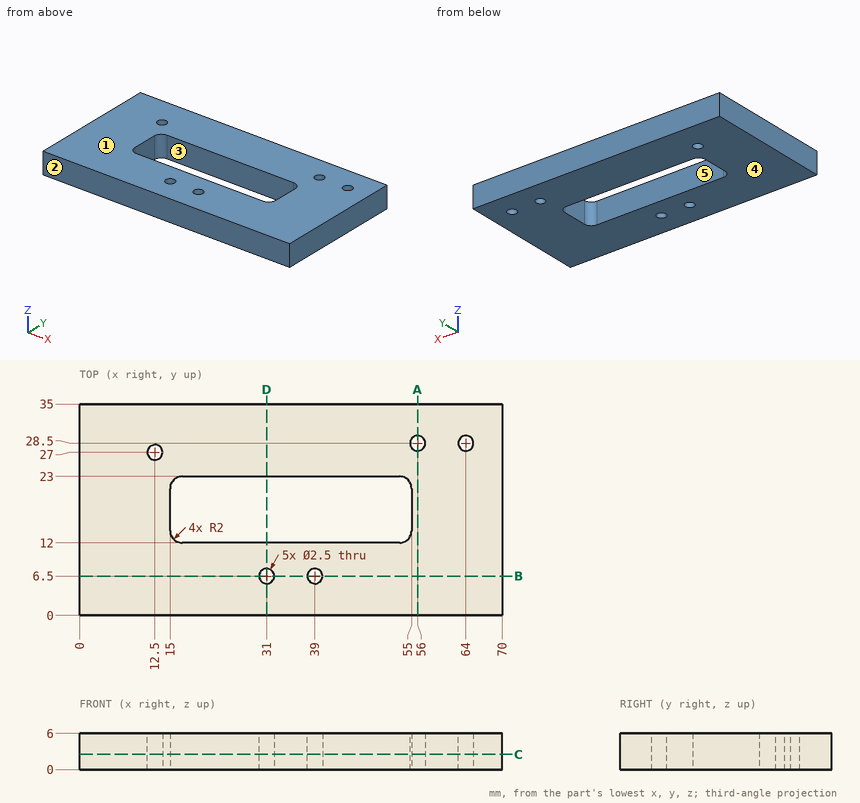
Drawing for the job (mm, zero at the part's lowest x, y, z). A direction names the side the tool comes from. Coordinates: 2 decimals unless noted, no trailing zeros. Order: outer loops, then holes, each group sorted by start corner. A loop starts at its lowest first (then second) coordinate and runs counter-clockwise, first axis right, second up. Notation, with made-up numbers: (28, 55.5) -> (49, 55.5) arc R29 ccw to (49, 90.5) -> close; hole circle Ø2 at (5.5, 65.5). An arc over 180 degrees is marked (long way). Return JSON: item names as keys, results as strings.
Item 1: Mould opens along Y. For the marked faces 1, 2 and 3 say: pulls with the +Y half, pulls with the -Y half, needs draft (parallel to the pull), parting line crosses it, or undercut.
Model answer:
{"face 1": "needs draft", "face 2": "pulls with the -Y half", "face 3": "undercut"}
Item 2: Slice it at C-C (z = 2.5). Write the cut outline in (x, y).
Model answer:
{"outline": "(0, 0) -> (70, 0) -> (70, 35) -> (0, 35) -> close; hole circle Ø2.5 at (12.5, 27); hole (15, 14) arc R2 ccw to (17, 12) -> (53, 12) arc R2 ccw to (55, 14) -> (55, 21) arc R2 ccw to (53, 23) -> (17, 23) arc R2 ccw to (15, 21) -> close; hole circle Ø2.5 at (31, 6.5); hole circle Ø2.5 at (39, 6.5); hole circle Ø2.5 at (56, 28.5); hole circle Ø2.5 at (64, 28.5)"}
Item 3: 3-axis set-ups, long thin cutter, end or side, ignore diameter. For the marked faces 4 and 5: which of +Z, -Z, +X, -X, +Y, -Y reach the whole face in a straight line?
Model answer:
{"face 4": "-Z, +X, -X, +Y, -Y", "face 5": "+Z, -Z"}
Item 4: Pin check, flat tips, straight feed: P1, Ø2, axis at x = 56, y = 28.5, coming from the +Z side; P2, Ø3, axis at x = 64, y = 28.5, coming from the +Z side. Stop position of each tip, or through.
Model answer:
{"P1": "passes through", "P2": "stops at z = 6"}
Item 5: Wall check: line 1 along Y through (x, z) = (31, 3.7); line 2 along X through (y, z) = (7, 1.5); line 3 along Y through (x, z) = (24.5, 0.75). Give the ranges that are in metal, low to high. Write a range as from..to.
Model answer:
{"line 1": "y = 0..5.25, 7.75..12, 23..35", "line 2": "x = 0..29.85, 32.15..37.85, 40.15..70", "line 3": "y = 0..12, 23..35"}
Item 6: Slice it at D-D (x = 31). Write the cut outline in (y, z), then the cut area to 3 significant figures.
Model answer:
{"outline": "(0, 0) -> (5.25, 0) -> (5.25, 6) -> (0, 6) -> close; (7.75, 0) -> (12, 0) -> (12, 6) -> (7.75, 6) -> close; (23, 0) -> (35, 0) -> (35, 6) -> (23, 6) -> close", "area": "129 mm²"}
Item 7: Slice it at A-A (x = 56). Write the cut outline in (y, z), then the cut area to 3 significant figures.
Model answer:
{"outline": "(0, 0) -> (27.25, 0) -> (27.25, 6) -> (0, 6) -> close; (29.75, 0) -> (35, 0) -> (35, 6) -> (29.75, 6) -> close", "area": "195 mm²"}
Item 8: Slice it at B-B (y = 6.5). Write the cut outline in (x, z).
Model answer:
{"outline": "(0, 0) -> (29.75, 0) -> (29.75, 6) -> (0, 6) -> close; (32.25, 0) -> (37.75, 0) -> (37.75, 6) -> (32.25, 6) -> close; (40.25, 0) -> (70, 0) -> (70, 6) -> (40.25, 6) -> close"}
